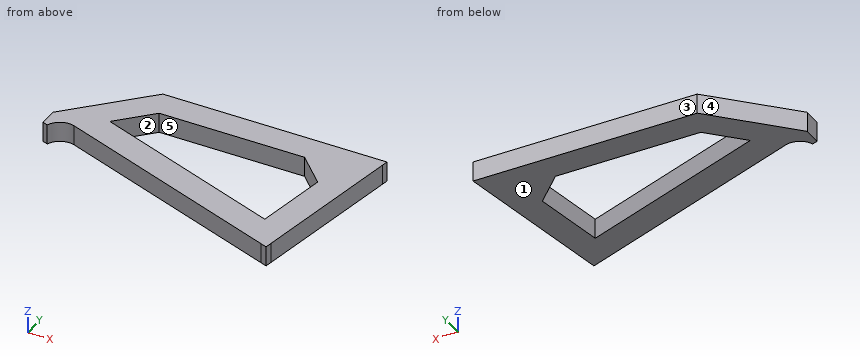
from build123d import *

# Parameters (mm, degrees)
BOSS_EXTRUDE2_DEPTH = 18


with BuildPart() as part:
    # Sketch5 → Boss-Extrude2 (new body)
    with BuildSketch(Plane.XY):
        with BuildLine():
            ThreePointArc((-239.737512556, -72.369347264), (-251.207088632, -72.87011977), (-258.963204018, -81.334434426))
            Line((-258.963204018, -81.334434426), (-263.661667122, -79.624333709))
            Line((-263.661667122, -79.624333709), (-263.661667122, -65.732734934))
            Line((-263.661667122, -65.732734934), (-263.661667122, -63.661667122))
            Line((-263.661667122, -63.661667122), (-262.197201028, -62.197201028))
            Line((-262.197201028, -62.197201028), (-201.464466094, -1.464466094))
            Line((-201.464466094, -1.464466094), (-200, 0))
            Line((-200, 0), (-197.928932188, 0))
            Line((-197.928932188, 0), (-5.958767963, 0))
            Line((-5.958767963, 0), (0, 0))
            Line((0, 0), (-1.034729198, -5.868240888))
            Line((-1.034729198, -5.868240888), (-25.414317908, -144.131759112))
            Line((-25.414317908, -144.131759112), (-26.449047106, -150))
            Line((-26.449047106, -150), (-32.04845739, -147.961981327))
            Line((-32.04845739, -147.961981327), (-239.737512556, -72.369347264))
        make_face()
        Polygon((-218.235614695, -53.590953754), (-45.895594942, -116.317591117), (-34.321629376, -50.678370624), (-60, -25), (-189.644660941, -25), align=None, mode=Mode.SUBTRACT)
    extrude(amount=BOSS_EXTRUDE2_DEPTH)


solid = part.part
For this review, take the finished solid that the model builds, in its own axes (mm). Face numbers are marked on the shaded views. A direction names the side the tool comes from. Give positions to 0.01 mm unless a question says otherwise; leave off trailing zeros. Loops run counter-clockwise (first coordinate to the right, second up) from the corner with the lowest first, then second, coordinate; pieces in that order, holes last. Notation, with made-up numbers: M -14,-28 L 16,-28 A9 cw 16,-21 Z; hole C -0.75,42 d4. An arc over 180 degrees is marked long. Put each result on its own line as item: value. Start each with the question number.
(1) The part is to be moulded in two halves that separate along Y. For the marked faces 1, 2 and 3, say which applies: +Y half, -Y half, draft (parallel to the pull), parting line (faces both ways), or undercut.
(2) Add section B-B, the plane x = -196. Write out the cut boundary in (y, z), then the cut area to 3 significant figures.
(3) Machinability: for the marked faces 4 and 5, which of the approach directions +Z, -Z, +X, -X, +Y, -Y give a long, thin tool a straight path to every point of the face, cutting with its end or side? Answer none if there is none.
(4) Wall thickness on L1, parallel to X at y = -47, z = 9.75; L2, parallel to Y at x = -68.5, z = 8; L3, parallel to Y at x = -46.5, z = 10: over which ranges is each line inside the solid? List them lowest first.
(5) Add section A-A, the plane y = -113.5. Write out the cut boundary in (x, z), then the cut area to 3 significant figures.
(6) Add section D-D, the plane y = -134.5. Write out the cut boundary in (x, z), then the cut area to 3 significant figures.
(7) For pin 1 (1.5 mm diameter, centred on x = -128, z = 2.5, fed in from -Y); pin 2 (1.5 mm diameter, centred on y = -78, z = 15, fed in from +X); pin 3 (10 mm diameter, centred on y = -52.5, z = 13.5, fed in from -X), all flat-tipped, find the tip position at first contact; note any pin that passes through.
(8) Add section C-C, the plane z = 3.5. Write out the cut boundary in (x, y).
Result:
1. face 1: draft
1. face 2: undercut
1. face 3: +Y half
2. outline: M -88.29,0 L -61.68,0 L -61.68,18 L -88.29,18 Z; M -31.36,0 L 0,0 L 0,18 L -31.36,18 Z
2. area: 1,040 mm^2
3. face 4: +Z, -Z, -X, +Y
3. face 5: +Z, -Z
4. L1: x = -247 to -211.64, -38 to -8.29
4. L2: y = -134.69 to -108.09, -25 to 0
4. L3: y = -142.7 to -116.1, -38.5 to 0
5. outline: M -126.73,0 L -53.64,0 L -53.64,18 L -126.73,18 Z; M -45.4,0 L -20.01,0 L -20.01,18 L -45.4,18 Z
5. area: 1,770 mm^2
6. outline: M -69.03,0 L -23.72,0 L -23.72,18 L -69.03,18 Z
6. area: 816 mm^2
7. pin 1: stops at y = -113.31
7. pin 2: stops at x = -13.62
7. pin 3: stops at x = -257.5
8. outline: M -263.66,-79.62 L -258.96,-81.33 A15 cw -239.74,-72.37 L -26.45,-150 L 0,0 L -200,0 L -263.66,-63.66 Z; hole M -218.24,-53.59 L -45.9,-116.32 L -34.32,-50.68 L -60,-25 L -189.64,-25 Z
